Autodesk Inventor part; units mm, degrees
ref_plane "YZ Plane" through (0, 0, 0) normal (1, 0, 0) x (0, 1, 0)
ref_plane "XZ Plane" through (0, 0, 0) normal (0, 1, 0) x (-1, 0, 0)
ref_plane "XY Plane" through (0, 0, 0) normal (0, 0, 1) x (1, 0, 0)
sketch "Skizze1" plane through (0, 0, 0) normal (0, 1, 0) x (-1, 0, 0)
  circle A0 centre (0, 0) radius 200
  dimension "d0" = 400
extrude "Extrusion1" add sketch "Skizze1" along normal mid plane 50
sketch "Skizze2" plane through (0, 25, 0) normal (0, 1, 0) x (1, 0, 0)
  circle A0 centre (0, 0) radius 200
hole "Bohrung1" at (0, 25, 0) direction (0, -1, 0) diameter 350 depth 15
mirror "Spiegeln1" about plane through (0, 0, 0) normal (0, 1, 0) of "Bohrung1"
sketch "Skizze3" plane through (0, 10, 0) normal (0, 1, 0) x (1, 0, 0)
  circle A0 centre (0, 0) radius 75
  dimension "d11" = 150
extrude "Extrusion2" add sketch "Skizze3" along normal blind 50
sketch "Skizze4" plane through (0, 60, 0) normal (0, 1, 0) x (1, 0, 0)
  circle A0 centre (0, 0) radius 75
hole "Bohrung2" at (0, 60, 0) direction (0, -1, 0) diameter 28 depth 70
sketch "Skizze7" plane through (0, -10, 0) normal (0, -1, 0) x (1, 0, 0)
  circle A0 centre (0, -48.21) radius 15
  point P0 (0, 0)
  dimension "d46" = 30
  dimension "d50" = 48.21
extrude "Extrusion3" add sketch "Skizze7" along normal blind 10
properties part number "rad" material "Gold"
Read the model definition and answer for the solid it produces. Units are mm, in the model's axes. A direction names the side the tool comes from. Coordinates: 2 decimals unless noted, no trailing zeros. Order: outer loops, then holes, each group sorted by start corner. A loop starts at its lowest first (then second) coordinate and runs counter-clockwise, first axis right, second up. Notation, with made-up numbers: M 78,89 L 88,89 A20 ccw 88,116 Z; hole C 15.25,59 d8. An arc over 180 degrees is marked long. Put each result on its own line as item: value. Start each with the question number.
Item 1: Section D-D, the plane y = 52 is taken. Determine the outline of the cut face in (x, z).
Item 2: Section A-A, the plane z = 0 is taken. Determine the outline of the cut face in (x, y), plus the area to 3 significant figures.
Item 3: Section B-B, the plane x = 0 is taken. Determine the outline of the cut face in (y, z).
Item 4: Given pin 1 Ø6 at (x, y) = (5.5, 39) entering from -Z; pin 2 Ø4 at (y, z) = (-2, -71) entering from -X; pin 3 Ø15 at (x, z) = (6.5, -54) entering from -Y, each flat-ended and moving along its own axis, determine where each tip first touches the part or whether it passes through.
Item 5: Section C-C, the plane z = -48.21 is taken. Determine the outline of the cut face in (x, y), plus the area to 3 significant figures.
Item 6: Consider probe 1 along Z at (x, y) = (0, 15.25); probe 2 along Z at (x, y) = (0, -16); probe 3 along Z at (x, y) = (0, 29). Determine where each line is inside the solid, lowest interval first. Write a range as [from, to].
Item 7: For faces 1 (the face through (0, -20, -48)), 2 (the face through (-118.273, 17.395, -128.982)), 3 (the face through (5.362, 24.51, 12.932)), determine the directions among +Z, -Z, +X, -X, +Y, -Y from which every point of the face is accessible in a straight line to the end or side of a thin tool.
Item 8: The mould has two halves that part along Z. Classify faces 4 (the face through (-1.953, -14.93, -63.082)), 5 (the face through (1, -25, -177)), 6 (the face through (-190.764, -0.35, -60.075)): +Z half, -Z half, draft (parallel to the pull), parting line (faces both ways), or undercut.
Computed:
1. outline: C 0,0 d150; hole C 0,0 d28
2. outline: M -200,-25 L -175,-25 L -175,-10 L -14,-10 L -14,60 L -75,60 L -75,10 L -175,10 L -175,25 L -200,25 Z; M 14,-10 L 175,-10 L 175,-25 L 200,-25 L 200,25 L 175,25 L 175,10 L 75,10 L 75,60 L 14,60 Z
2. area: 15,000 mm2
3. outline: M -25,-200 L 25,-200 L 25,-175 L 10,-175 L 10,-75 L 60,-75 L 60,-14 L -10,-14 L -10,-33.21 L -20,-33.21 L -20,-63.21 L -10,-63.21 L -10,-175 L -25,-175 Z; M -25,175 L -10,175 L -10,14 L 60,14 L 60,75 L 10,75 L 10,175 L 25,175 L 25,200 L -25,200 Z
4. pin 1: stops at z = -74.96
4. pin 2: stops at x = -187.72
4. pin 3: stops at y = -20
5. outline: M -194.1,-25 L -168.23,-25 L -168.23,-10 L -15,-10 L -15,-20 L 15,-20 L 15,-10 L 168.23,-10 L 168.23,-25 L 194.1,-25 L 194.1,25 L 168.23,25 L 168.23,10 L 57.45,10 L 57.45,60 L -57.45,60 L -57.45,10 L -168.23,10 L -168.23,25 L -194.1,25 Z
5. area: 15,400 mm2
6. probe 1: z = [-200, -175], [-75, -14], [14, 75], [175, 200]
6. probe 2: z = [-200, -175], [-63.21, -33.21], [175, 200]
6. probe 3: z = [-75, -14], [14, 75]
7. face 1: -Y
7. face 2: +Y
7. face 3: +Y, -Y
8. face 4: undercut
8. face 5: draft
8. face 6: parting line
